Read the model definition and answer for the solid it produces. Units are mm, in the model's axes. A direction names the side the tool comes from. Coordinates: 2 decimals unless noted, no trailing zeros. Order: outer loops, then holes, each group sorted by start corner. A loop starts at its lowest first (then second) coordinate and runs counter-clockwise, first axis right, second up. Notation, with made-up numbers: (83.5, 79.25) -> (112.5, 79.25) arc R4 ccw to (112.5, 84.25) -> close; hole circle Ø1 at (17, 58.5). An arc over 180 degrees is marked (long way). Answer in a Markdown table with one row per item.
from build123d import *

# Parameters (mm, degrees)
SKETCH_2_R          = 27
CUT_EXTRUDE_1_DEPTH = 66
SKETCH_3_R          = 28.9
CUT_EXTRUDE_2_DEPTH = 11
SKETCH_4_R          = 23
CUT_EXTRUDE_3_DEPTH = 94.145048178
FILLET_1_R          = 1
FILLET_3_R          = 1


with BuildPart() as part:
    # 草圖1 → 旋轉1 (revolve)
    with BuildSketch(Plane.XY, mode=Mode.PRIVATE) as revolve_1_sk:
        Polygon((0, 0), (36, 0), (31.25, 89), (0, 89), align=None)
    revolve(revolve_1_sk.sketch.rotate(Axis((0, 89, 0), (0, -1, 0)), 180), axis=Axis((0, 89, 0), (0, -1, 0)))

    # 草圖2 → 除料-伸長1 (cut)
    with BuildSketch(Plane(origin=(0, 89, 0), x_dir=(1, 0, 0), z_dir=(0, 1, 0))):
        with Locations(Location((0, 0, 0), (0, 0, 180))):
            Circle(SKETCH_2_R)
    extrude(amount=-CUT_EXTRUDE_1_DEPTH, mode=Mode.SUBTRACT)

    # 草圖3 → 除料-伸長2 (cut)
    with BuildSketch(Plane.XZ):
        Circle(SKETCH_3_R)
    extrude(amount=-CUT_EXTRUDE_2_DEPTH, mode=Mode.SUBTRACT)

    # 草圖4 → 除料-伸長3 (cut, through all)
    with BuildSketch(Plane.XZ.offset(-11)):
        Circle(SKETCH_4_R)
    extrude(amount=-CUT_EXTRUDE_3_DEPTH, mode=Mode.SUBTRACT)

    # 圓角1
    fillet_1_edges = [part.edges().sort_by_distance(p)[0] for p in [
        (27, 89, 0),
    ]]
    fillet(fillet_1_edges, radius=FILLET_1_R)

    # 圓角3
    fillet_3_edges = [part.edges().sort_by_distance(p)[0] for p in [
        (-23, 23, 0),
        (-23, 11, 0),
    ]]
    fillet(fillet_3_edges, radius=FILLET_3_R)


solid = part.part
Q1. The part is cut by section C-C (y = 76). Write down the section's boundary in (x, z), then the cut area to 3 significant figures.
Outcome:
| item | result |
|---|---|
| outline | circle Ø63.89 at (0, 0); hole circle Ø54 at (0, 0) |
| area | 915 mm² |
Q2. For a pull along X with two mould halves and no side action, classify faces 1 (the face through (24.1, 23, -1.9)), 2 (the face through (15.536, 5.423, 24.369)), 3 (the face through (4.373, 45.123, -33.306)), 4 (the face through (26, 89, -12)) as pulls with the +X half, pulls with the -X half, needs draft (parallel to the pull), parting line crosses it, or undercut.
Outcome:
| item | result |
|---|---|
| face 1 | undercut |
| face 2 | undercut |
| face 3 | parting line crosses it |
| face 4 | needs draft |
Q3. For faces 5 (the face through (4, 11, 24)), 6 (the face through (5.85, 55.96, -26.36)), 7 (the face through (-2.994, 16.93, 22.804)), determine the directions among +Z, -Z, +X, -X, +Y, -Y from which every point of the face is accessible in a straight line to the end or side of a thin tool.
Outcome:
| item | result |
|---|---|
| face 5 | -Y |
| face 6 | +Y |
| face 7 | +Y, -Y |
Q4. The part is cut by section D-D (y = 54.5). Write down the section's boundary in (x, z).
Outcome:
| item | result |
|---|---|
| outline | circle Ø66.18 at (0, 0); hole circle Ø54 at (0, 0) |
Q5. Given pin 1 (4 mm diameter, centred on x = 15.5, y = 12.5, fed in from -Z); pin 2 (12 mm diameter, centred on y = 76, z = 9, fed in from +X); pin 3 (12 mm diameter, centred on x = 2.5, y = 25, fed in from -Z), each flat-ended and moving along its own axis, determine where each tip first touches the part or whether it passes through.
Outcome:
| item | result |
|---|---|
| pin 1 | z = -32.66 |
| pin 2 | x = 31.88 |
| pin 3 | z = -34.96 |
Q6. The part is cut by section B-B (x = 0). Write down the section's boundary in (y, z), then the cut area to 3 significant figures.
Outcome:
| item | result |
|---|---|
| outline | (0, -36) -> (89, -31.25) -> (89, -28) arc R1 ccw to (88, -27) -> (23, -27) -> (23, -24) arc R1 ccw to (22, -23) -> (12, -23) arc R1 ccw to (11, -24) -> (11, -28.9) -> (0, -28.9) -> close; (0, 28.9) -> (11, 28.9) -> (11, 24) arc R1 ccw to (12, 23) -> (22, 23) arc R1 ccw to (23, 24) -> (23, 27) -> (88, 27) arc R1 ccw to (89, 28) -> (89, 31.25) -> (0, 36) -> close |
| area | 1,230 mm² |
Q7. The part is cut by section A-A (z = 0). Write down the section's boundary in (x, y), then the cut area to 3 significant figures.
Outcome:
| item | result |
|---|---|
| outline | (-36, 0) -> (-28.9, 0) -> (-28.9, 11) -> (-24, 11) arc R1 ccw to (-23, 12) -> (-23, 22) arc R1 ccw to (-24, 23) -> (-27, 23) -> (-27, 88) arc R1 ccw to (-28, 89) -> (-31.25, 89) -> close; (23, 12) arc R1 ccw to (24, 11) -> (28.9, 11) -> (28.9, 0) -> (36, 0) -> (31.25, 89) -> (28, 89) arc R1 ccw to (27, 88) -> (27, 23) -> (24, 23) arc R1 ccw to (23, 22) -> close |
| area | 1,230 mm² |
Q8. Consider line 1 (Y direction, x = -28, z = 3); line 2 (Z direction, x = -16, y = 83); line 3 (Z direction, x = 0, y = 4.75). Determine where each line is inside the solid, lowest interval first.
Outcome:
| item | result |
|---|---|
| line 1 | 11 to 89 |
| line 2 | -27.22 to -21.75, 21.75 to 27.22 |
| line 3 | -35.75 to -28.9, 28.9 to 35.75 |
